Here's how the part is built. I have some questions about the finished solid (model axes, mm). Face numbers are marked on the shaded views. A direction names the side the tool comes from. Round coordinates to 2 decimals unless told otherwise and drop trailing zeros. Order: outer loops, then holes, each group sorted by start corner. A loop starts at its lowest first (then second) coordinate and runs counter-clockwise, first axis right, second up. Notation, with made-up numbers: (69.25, -21) - (86.25, -21) arc R17 cw to (86.25, 6) - close; hole circle Ø1 at (72, 65). An arc over 180 degrees is marked (long way). Answer as a JSON object with one key per item and string values.
```python
from build123d import *

# Parameters (mm, degrees)
SKIZZE1_R                       = 18.5
AUFSATZ_LINEAR_AUSTRAGEN1_DEPTH = 27
SKIZZE2_R                       = 17.5
AUFSATZ_LINEAR_AUSTRAGEN2_DEPTH = 29
SKIZZE3_R                       = 1.5
SCHNITT_LINEAR_AUSTRAGEN1_DEPTH = 10
SKIZZE4_R                       = 6
AUFSATZ_LINEAR_AUSTRAGEN3_DEPTH = 6
SKIZZE5_R                       = 3
AUFSATZ_LINEAR_AUSTRAGEN4_DEPTH = 15
SKIZZE6_W                       = 6
SKIZZE6_H                       = 1
SCHNITT_LINEAR_AUSTRAGEN2_DEPTH = 12


with BuildPart() as part:
    # Skizze1 → Aufsatz-Linear austragen1 (new body)
    with BuildSketch(Plane(origin=(0, 0, 0), x_dir=(1, 0, 0), z_dir=(0, 1, 0))):
        with Locations(Location((0, 0, 0), (0, 0, 270))):
            Circle(SKIZZE1_R)
    extrude(amount=AUFSATZ_LINEAR_AUSTRAGEN1_DEPTH)

    # Skizze2 → Aufsatz-Linear austragen2 (add)
    with BuildSketch(Plane(origin=(0, 27, 0), x_dir=(1, 0, 0), z_dir=(0, 1, 0))):
        with Locations(Location((0, 0, 0), (0, 0, 90))):
            Circle(SKIZZE2_R)
    extrude(amount=AUFSATZ_LINEAR_AUSTRAGEN2_DEPTH)

    # Skizze3 → Schnitt-Linear austragen1 (cut)
    with BuildSketch(Plane.XZ):
        with Locations(Location((-15.5, 0, 0), (0, 0, 270))):
            Circle(SKIZZE3_R)
        with Locations(Location((15.5, 0, 0), (0, 0, 270))):
            Circle(SKIZZE3_R)
        with Locations(Location((7.75, 13.423393759, 0), (0, 0, 270))):
            Circle(SKIZZE3_R)
        with Locations(Location((-7.75, 13.423393759, 0), (0, 0, 270))):
            Circle(SKIZZE3_R)
        with Locations(Location((-7.75, -13.423393759, 0), (0, 0, 270))):
            Circle(SKIZZE3_R)
        with Locations(Location((7.75, -13.423393759, 0), (0, 0, 270))):
            Circle(SKIZZE3_R)
    extrude(amount=-SCHNITT_LINEAR_AUSTRAGEN1_DEPTH, mode=Mode.SUBTRACT)

    # Skizze4 → Aufsatz-Linear austragen3 (add)
    with BuildSketch(Plane.XZ):
        with Locations(Location((0, 7, 0), (0, 0, 90))):
            Circle(SKIZZE4_R)
    extrude(amount=AUFSATZ_LINEAR_AUSTRAGEN3_DEPTH)

    # Skizze5 → Aufsatz-Linear austragen4 (add)
    with BuildSketch(Plane.XZ.offset(6)):
        with Locations(Location((0, 7, 0), (0, 0, 270))):
            Circle(SKIZZE5_R)
    extrude(amount=AUFSATZ_LINEAR_AUSTRAGEN4_DEPTH)

    # Skizze6 → Schnitt-Linear austragen2 (cut)
    with BuildSketch(Plane.XZ.offset(21)):
        with Locations((0, 10)):
            Rectangle(SKIZZE6_W, SKIZZE6_H)
    extrude(amount=-SCHNITT_LINEAR_AUSTRAGEN2_DEPTH, mode=Mode.SUBTRACT)


solid = part.part
```
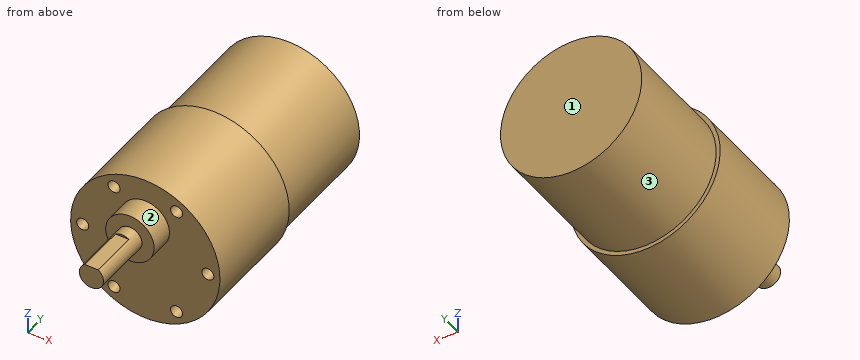
1. Imagine slicing it at C-C (z = 5). List the corners of the cut face in (x, y) for me, plus the area to 3 significant figures.
Responses:
{"outline": "(-17.81, 0) - (-5.66, 0) - (-5.66, -6) - (-2.24, -6) - (-2.24, -21) - (2.24, -21) - (2.24, -6) - (5.66, -6) - (5.66, 0) - (17.81, 0) - (17.81, 27) - (16.77, 27) - (16.77, 56) - (-16.77, 56) - (-16.77, 27) - (-17.81, 27) - close", "area": "2,070 mm2"}
2. If I drill on L1, parallel to X at y = 6.5, z = 0; L2, parallel to Z at x = 7, y = 5; L3, parallel to Y at x = 2, z = 2, over which ranges is the centre line in solid material (lowest first)? Write a range as [from, to].
Responses:
{"L1": "[-18.5, -17], [-14, 14], [17, 18.5]", "L2": "[-17.12, -14.72], [-12.12, 12.12], [14.72, 17.12]", "L3": "[-6, 56]"}
3. Imagine slicing it at B-B (x = 0). List the corners of the cut face in (y, z) for me, plus the area to 3 significant figures.
Responses:
{"outline": "(-21, 4) - (-6, 4) - (-6, 1) - (0, 1) - (0, -18.5) - (27, -18.5) - (27, -17.5) - (56, -17.5) - (56, 17.5) - (27, 17.5) - (27, 18.5) - (0, 18.5) - (0, 13) - (-6, 13) - (-6, 10) - (-9, 10) - (-9, 9.5) - (-21, 9.5) - close", "area": "2,170 mm2"}
4. For the marked faces 1, 2 and 3, which set-ups out of +Z, -Z, +X, -X, +Y, -Y let a thin tool reach every point of the face, with its end or its side?
Responses:
{"face 1": "+Z, -Z, +X, -X, +Y", "face 2": "-Y", "face 3": "+Y"}
5. For P1, Ø1.5, axis at x = 8, z = -12.5, coming from the -Y side; P2, Ø3, axis at y = 12.5, z = 3.5, coming from the -X side; P3, Ø0.9, axis at x = -15.5, z = 0, coming from the -Y side, each with a flat end and sliding along its axis, tell me the tip position at first contact or that it passes through.
Responses:
{"P1": "y = 0", "P2": "x = -18.39", "P3": "y = 10"}
6. Imagine slicing it at D-D (y = 14.5). List the corners of the cut face in (x, z) for me.
Responses:
{"outline": "circle Ø37 at (0, 0)"}
7. Imagine slicing it at A-A (y = 2.5). List the corners of the cut face in (x, z) for me, plus the area to 3 significant figures.
Responses:
{"outline": "circle Ø37 at (0, 0); hole circle Ø3 at (-15.5, 0); hole circle Ø3 at (-7.75, -13.42); hole circle Ø3 at (-7.75, 13.42); hole circle Ø3 at (7.75, -13.42); hole circle Ø3 at (7.75, 13.42); hole circle Ø3 at (15.5, 0)", "area": "1,030 mm2"}
